```python
from build123d import *

# Parameters (mm, degrees)
F0_R          = 50.8
F1_DEPTH      = 203.2
F2_R          = 6.35
F3_DEPTH      = 127
F3_DEPTH_BACK = 127
F4_R          = 38.1
F5_DEPTH      = 177.8


with BuildPart() as f1:
    # F0 (on Top) → F1 (new body)
    with BuildSketch(Plane.XY):
        Circle(F0_R)
    extrude(amount=F1_DEPTH)

    # F2 (on Right) → F3 (join, two sides)
    with BuildSketch(Plane.YZ) as f3_sk:
        with Locations((0, 165.1)):
            Circle(F2_R)
    extrude(amount=F3_DEPTH)
    extrude(f3_sk.sketch, amount=-F3_DEPTH_BACK)

    # F4 (on face) → F5 (cut)
    with BuildSketch(Plane(origin=(0, 0, 0), x_dir=(1, 0, 0), z_dir=(0, 0, -1))):
        Circle(F4_R)
    extrude(amount=-F5_DEPTH, mode=Mode.SUBTRACT)


solid = f1.part
```
CAD build for the part. Positions are in the model's coordinates, mm. A direction names the side the tool comes from. Round coordinates to 2 decimals unless told otherwise and drop trailing zeros. Order: outer loops, then holes, each group sorted by start corner. A loop starts at its lowest first (then second) coordinate and runs counter-clockwise, first axis right, second up. Notation, with made-up numbers: (61.25, 41.25) - (114.25, 41.25) arc R15 ccw to (114.25, 67.25) - close; hole circle Ø1 at (87.25, 47.5). An arc over 180 degrees is marked (long way). Answer as CSV lines item,"result". Start each with the question number.
1. Saw through at B-B, the plane y = 0. Write the cut outline in (x, z).
2. Tool access for faces 4 (the face through (-88.16, -1.38, 158.9)), 5 (the face through (-30.235, 23.183, 87.655)), 6 (the face through (127, 0, 165)): list every direction of +Z, -Z, +X, -X, +Y, -Y with a clear straight run to the whole face (end or side of a thin tool).
3. Saw through at A-A, the plane z = 165.1. Write the cut outline in (x, y).
4. Saw through at D-D, the plane z = 28. Write the cut outline in (x, y), and give its area (3 significant figures).
5. Pin check, flat tips, straight feed: pin 1 (2 mm diameter, centred on x = 71, z = 171.5, fed in from +Y); pin 2 (6 mm diameter, centred on x = -22.5, z = 129, fed in from +Y); pin 3 (3 mm diameter, centred on y = -27, z = 182.5, fed in from +X). Stop position of each tip, or through.
6. Saw through at C-C, the plane x = 0. Write the cut outline in (y, z), and give its area (3 significant figures).
7. Drill centre lines: L1, parallel to Y at x = 0, z = 44.5; L2, parallel to Y at x = -22.5, z = 55. Where is each one in solid material? Low to high. Write a range as [from, to].
8. Pull direction Y, two halves, no side cores. Call faces 1 (the face through (88.16, -1.38, 158.9)), 2 (the face through (-1, -1, 177.8)), 3 (the face through (-127, 0, 165)): +Y half, -Y half, draft (parallel to the pull), parting line (faces both ways), or undercut.
Model answer:
1,outline,"(-127, 158.75) - (-50.8, 158.75) - (-50.8, 0) - (-38.1, 0) - (-38.1, 177.8) - (38.1, 177.8) - (38.1, 0) - (50.8, 0) - (50.8, 158.75) - (127, 158.75) - (127, 171.45) - (50.8, 171.45) - (50.8, 203.2) - (-50.8, 203.2) - (-50.8, 171.45) - (-127, 171.45) - close"
2,face 4,"-X"
2,face 5,"-Z"
2,face 6,"+Z, -Z, +X, +Y, -Y"
3,outline,"(-127, -6.35) - (-50.4, -6.35) arc R50.8 ccw to (50.4, -6.35) - (127, -6.35) - (127, 6.35) - (50.4, 6.35) arc R50.8 ccw to (-50.4, 6.35) - (-127, 6.35) - close; hole circle Ø76.2 at (0, 0)"
4,outline,"circle Ø101.6 at (0, 0); hole circle Ø76.2 at (0, 0)"
4,area,"3,550 mm²"
5,pin 1,"stops at y = 3.34"
5,pin 2,"stops at y = 46.91"
5,pin 3,"stops at x = 43.94"
6,outline,"(-50.8, 0) - (-38.1, 0) - (-38.1, 177.8) - (38.1, 177.8) - (38.1, 0) - (50.8, 0) - (50.8, 203.2) - (-50.8, 203.2) - close"
6,area,"7,100 mm²"
7,L1,"y = [-50.8, -38.1], [38.1, 50.8]"
7,L2,"y = [-45.55, -30.75], [30.75, 45.55]"
8,face 1,"parting line"
8,face 2,"undercut"
8,face 3,"draft"
